```python
from build123d import *

# Parameters (mm, degrees)
SKETCH1_W               = 44.958
SKETCH1_H               = 304.8
BOSS_EXTRUDE1_DEPTH     = 5.588
BOSS_EXTRUDE2_DEPTH     = 5.588
SKETCH3_W               = 121.412
SKETCH3_H               = 5.588
BOSS_EXTRUDE3_DEPTH     = 39.37
SKETCH8_W               = 5.588
SKETCH8_H               = 213.451350416
CUT_EXTRUDE4_DEPTH      = 1
CUT_EXTRUDE4_DEPTH_BACK = 133.588
SKETCH6_W               = 5.588
SKETCH6_H               = 12.7
CUT_EXTRUDE5_DEPTH      = 5.588
SKETCH4_3_W             = 6.35
SKETCH4_3_H             = 15.875
SKETCH4_3_H_2           = 5.588
SKETCH4_3_H_3           = 7.112
CUT_EXTRUDE6_DEPTH      = 5.588


with BuildPart() as part:
    # Sketch1 → Boss-Extrude1 (new body)
    with BuildSketch(Plane.XY):
        with Locations((-6.477, 3.048)):
            Rectangle(SKETCH1_W, SKETCH1_H)
        with BuildLine():
            Line((-3.302, 133.858), (-3.302, -143.002))
            Line((-3.302, -143.002), (3.302, -143.002))
            Line((3.302, -143.002), (3.302, 143.002))
            Line((3.302, 143.002), (-16.256, 143.002))
            Line((-16.256, 143.002), (-16.256, 136.398))
            Line((-16.256, 136.398), (-5.842, 136.398))
            ThreePointArc((-5.842, 136.398), (-4.045948776, 135.654051224), (-3.302, 133.858))
        make_face(mode=Mode.SUBTRACT)
    extrude(amount=BOSS_EXTRUDE1_DEPTH)

    # Sketch2 → Boss-Extrude2 (add)
    with BuildSketch(Plane(origin=(16.002, 0, 0), x_dir=(0, 0, -1), z_dir=(1, 0, 0))):
        Polygon((121.412, -47.752), (-5.588, -47.752), (-5.588, -149.352), (121.412, -149.352), (121.412, -136.652), (127, -136.652), (127, -119.718666667), (121.412, -119.718666667), (121.412, -107.018666667), (127, -107.018666667), (127, -90.085333333), (121.412, -90.085333333), (121.412, -77.385333333), (127, -77.385333333), (127, -60.452), (121.412, -60.452), align=None)
        with BuildLine():
            ThreePointArc((11.9, -106.092), (10.4, -107.592), (8.9, -106.092))
            Line((8.9, -106.092), (8.9, -101.012))
            ThreePointArc((8.9, -101.012), (10.4, -99.512), (11.9, -101.012))
            Line((11.9, -101.012), (11.9, -106.092))
        make_face(mode=Mode.SUBTRACT)
        with BuildLine():
            ThreePointArc((60.9, -106.092), (59.4, -107.592), (57.9, -106.092))
            Line((57.9, -106.092), (57.9, -101.012))
            ThreePointArc((57.9, -101.012), (59.4, -99.512), (60.9, -101.012))
            Line((60.9, -101.012), (60.9, -106.092))
        make_face(mode=Mode.SUBTRACT)
        with BuildLine():
            Line((8.9, -96.092), (8.9, -91.012))
            ThreePointArc((8.9, -91.012), (10.4, -89.512), (11.9, -91.012))
            Line((11.9, -91.012), (11.9, -96.092))
            ThreePointArc((11.9, -96.092), (10.4, -97.592), (8.9, -96.092))
        make_face(mode=Mode.SUBTRACT)
        with BuildLine():
            ThreePointArc((36.4, -101.092), (25.4, -112.092), (14.4, -101.092))
            Line((14.4, -101.092), (14.4, -96.012))
            ThreePointArc((14.4, -96.012), (25.4, -85.012), (36.4, -96.012))
            Line((36.4, -96.012), (36.4, -101.092))
        make_face(mode=Mode.SUBTRACT)
        with BuildLine():
            ThreePointArc((57.9, -91.012), (59.4, -89.512), (60.9, -91.012))
            Line((60.9, -91.012), (60.9, -96.092))
            ThreePointArc((60.9, -96.092), (59.4, -97.592), (57.9, -96.092))
            Line((57.9, -96.092), (57.9, -91.012))
        make_face(mode=Mode.SUBTRACT)
    extrude(amount=-BOSS_EXTRUDE2_DEPTH)

    # Sketch3 → Boss-Extrude3 (add)
    with BuildSketch(Plane.ZY.offset(-10.414)):
        with Locations((-60.706, -146.558)):
            Rectangle(SKETCH3_W, SKETCH3_H)
    extrude(amount=BOSS_EXTRUDE3_DEPTH)

    # Sketch8 → Cut-Extrude4 (cut, two sides)
    with BuildSketch(Plane.XY.offset(5.588)) as cut_extrude4_sk:
        Polygon((-28.956, -149.352), (10.414, -149.352), (10.414, -47.752), (10.414, 155.448), (-28.956, 155.448), align=None)
        with BuildLine():
            Line((-16.256, 136.398), (-16.256, 143.002))
            Line((-16.256, 143.002), (3.302, 143.002))
            Line((3.302, 143.002), (3.302, -143.002))
            Line((3.302, -143.002), (-3.302, -143.002))
            Line((-3.302, -143.002), (-3.302, 133.858))
            ThreePointArc((-3.302, 133.858), (-4.045948776, 135.654051224), (-5.842, 136.398))
            Line((-5.842, 136.398), (-16.256, 136.398))
        make_face(mode=Mode.SUBTRACT)
        Polygon((-54.223542679, -149.352), (-28.956, -149.352), (-28.956, 155.448), (10.414, 155.448), (10.414, 165.699350416), (-54.223542679, 165.699350416), align=None)
        with Locations((13.208, 58.973675208)):
            Rectangle(SKETCH8_W, SKETCH8_H)
    extrude(amount=CUT_EXTRUDE4_DEPTH, mode=Mode.SUBTRACT)
    extrude(cut_extrude4_sk.sketch, amount=-CUT_EXTRUDE4_DEPTH_BACK, mode=Mode.SUBTRACT)

    # Sketch6 → Cut-Extrude5 (cut)
    with BuildSketch(Plane.XY.offset(5.588)):
        with Locations((13.208, -54.102)):
            Rectangle(SKETCH6_W, SKETCH6_H)
        with Locations((13.208, -83.735333333)):
            Rectangle(SKETCH6_W, SKETCH6_H)
        with Locations((13.208, -113.368666667)):
            Rectangle(SKETCH6_W, SKETCH6_H)
        with Locations((13.208, -143.002)):
            Rectangle(SKETCH6_W, SKETCH6_H)
    extrude(amount=-CUT_EXTRUDE5_DEPTH, mode=Mode.SUBTRACT)

    # Sketch4<3> → Cut-Extrude6 (cut)
    with BuildSketch(Plane.XZ.offset(149.352)):
        with Locations((12.827, -100.7745)):
            Rectangle(SKETCH4_3_W, SKETCH4_3_H)
        with Locations((12.827, -72.1995)):
            Rectangle(SKETCH4_3_W, SKETCH4_3_H)
        with Locations((12.827, -43.6245)):
            Rectangle(SKETCH4_3_W, SKETCH4_3_H)
        with Locations((12.827, -15.0495)):
            Rectangle(SKETCH4_3_W, SKETCH4_3_H)
        with Locations((12.827, 2.794)):
            Rectangle(SKETCH4_3_W, SKETCH4_3_H_2)
        with Locations((12.827, -3.556)):
            Rectangle(SKETCH4_3_W, SKETCH4_3_H_3)
    extrude(amount=-CUT_EXTRUDE6_DEPTH, mode=Mode.SUBTRACT)


solid = part.part
```
The model under review builds one solid part; all positions refer to its coordinate system, in mm. A direction names the side the tool comes from. Give positions to 0.01 mm unless a question says otherwise; leave off trailing zeros. Write each loop counter-clockwise with the first axis right and the second up, starting at its lowest first coordinate (ties: lowest second). Pieces come first, ordered by that corner, then holes. Notation, with made-up numbers: (-34, -13.5) - (-11, -13.5) arc R14 cw to (-11, -6.5) - close; hole circle Ø7 at (28, 7). An arc over 180 degrees is marked (long way). Answer in a Markdown table with one row per item. Add a question column.
1. Tool access review of faces 1 (the flat face through (13, -77.385, 3)), 2 (the flat face through (13, -77.385, -124)), 3 (the flat face through (13, -94, -8.9)), 4 (the flat face through (13, -147, -64.262)): name each direction out of +Z, -Z, +X, -X, +Y, -Y from which nothing blocks a thin tool from reaching the whole face with its end or side.
2. We need section B-B on z = -25.4. Write out the cut boundary in (x, y).
3. Wall thickness on line 1 along Z through (x, y) = (13.7, -145); line 2 along Z through (x, y) = (13.2, -96); line 3 along Z through (x, y) = (10.75, -143): over which ranges is each line inside the solid? List them lowest first. Write a range as [from, to].
4. We need section C-C on z = -59.4. Write out the cut boundary in (x, y).
5. Draft analysis for pull direction Y (two halves, no side actions). For faces 5 (the cylindrical face through (13.25, -97.59, -10.43)), 6 (the flat face through (16.002, -98, -60)), 7 (the flat face through (13, -143.764, -101)), state which applies: +Y half, -Y half, draft (parallel to the pull), parting line (faces both ways), or undercut.
6. We need section A-A on z = -10.4. Write out the cut boundary in (x, y).
7. Insertion check: P1, Ø2, axis at x = 13.5, y = -118.5, coming from the +Z side; P2, Ø1.7, axis at x = 12.5, y = -147, coming from the +Z side; P3, Ø1.7, axis at x = 12, z = -124, coming from the -Y side. Each pin has a flat end and moves straight along its axis. Give the tip position at first contact, or say it passes through.
8. We need section D-D on x = 13.5. State how many separate pieces and enclosed holes the cut face has, then the cut area to 3 significant figures.
Ans:
| question | item | result |
|---|---|---|
| 1 | face 1 | +Z, +X, -X |
| 1 | face 2 | -Z, +X, -X |
| 1 | face 3 | +X, -X |
| 1 | face 4 | +X, -X, -Y |
| 2 | outline | (10.41, -149.35) - (16, -149.35) - (16, -112.09) - (10.41, -112.09) - close; (10.41, -85.01) - (16, -85.01) - (16, -47.75) - (10.41, -47.75) - close |
| 3 | line 1 | z = [-121.41, -108.71], [-92.84, -80.14], [-64.26, -51.56], [-35.69, -22.99] |
| 3 | line 2 | z = [-127, -60.9], [-57.9, -36.4], [-14.4, -11.9], [-8.9, 5.59] |
| 3 | line 3 | z = [-121.41, 0] |
| 4 | outline | (10.41, -149.35) - (16, -149.35) - (16, -107.59) - (10.41, -107.59) - close; (10.41, -99.51) - (16, -99.51) - (16, -97.59) - (10.41, -97.59) - close; (10.41, -89.51) - (16, -89.51) - (16, -47.75) - (10.41, -47.75) - close |
| 5 | face 5 | undercut |
| 5 | face 6 | draft |
| 5 | face 7 | -Y half |
| 6 | outline | (10.41, -143.76) - (16, -143.76) - (16, -107.59) - (10.41, -107.59) - close; (10.41, -99.51) - (16, -99.51) - (16, -97.59) - (10.41, -97.59) - close; (10.41, -89.51) - (16, -89.51) - (16, -47.75) - (10.41, -47.75) - close |
| 7 | P1 | stops at z = 0 |
| 7 | P2 | stops at z = -22.99 |
| 7 | P3 | stops at y = -136.65 |
| 8 | separate pieces | 1 |
| 8 | enclosed holes | 5 |
| 8 | area | 11,900 mm^2 |
